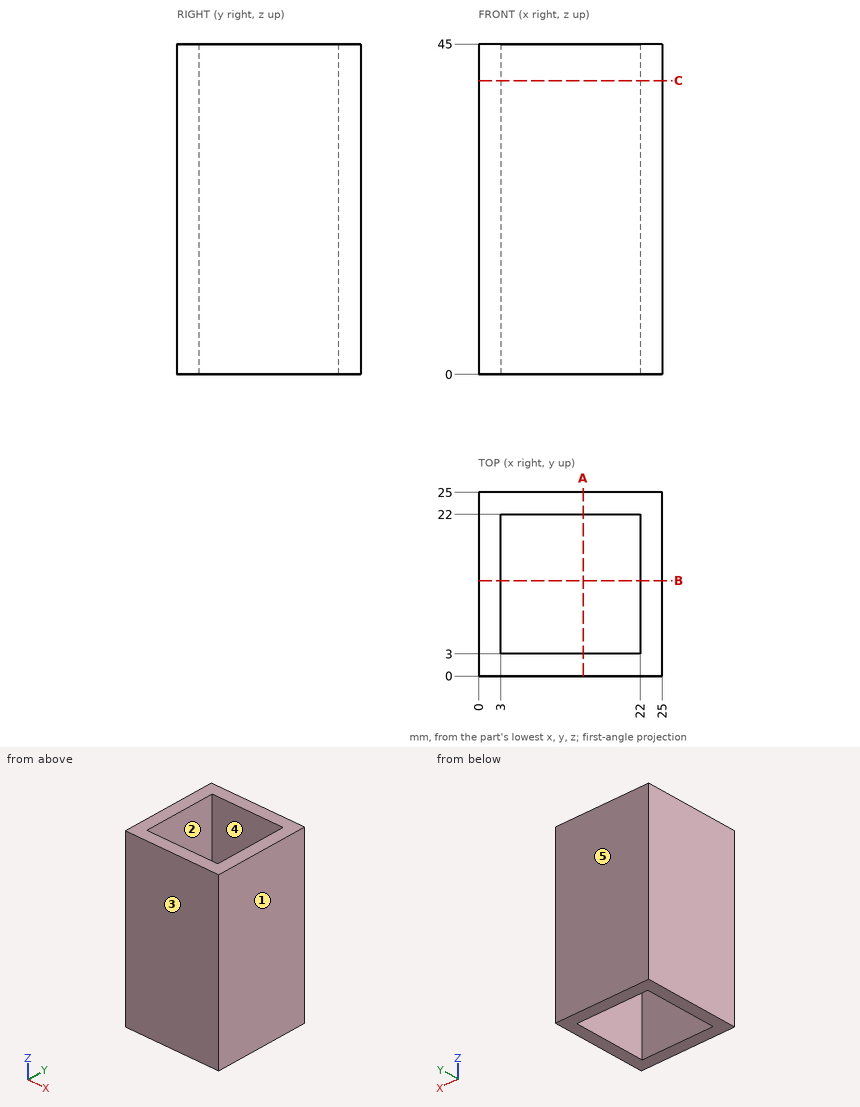
The drawing under review shows one solid part. Ordinate dimensions are in mm from its lowest x, y, z. A direction names the side the tool comes from. Round coordinates to 2 decimals unless told otherwise and drop trailing zeros. Loops run counter-clockwise (first coordinate to the right, second up) from the corner with the lowest first, then second, coordinate; pieces in that order, holes last. Notation, with made-up numbers: (-8, 86.5) - (47, 86.5) arc R37 cw to (47, 122.5) - close; hole circle Ø5 at (-25.75, 62.5). An arc over 180 degrees is marked (long way). One line per question, with ' | ' between items.
1. Draft analysis for pull direction Y (two halves, no side actions). For the marked faces 3, 4 and 5, state which applies: released by +Y, released by -Y, zero draft, split by the parting line, or undercut.
Results are:
face 3: released by -Y | face 4: undercut | face 5: released by +Y
2. For L1, parallel to Y at x = 8.75, z = 25.5, list the stretches that pass through material, from the lowest coordinate up. Write a range as [from, to].
Results are:
L1: y = [0, 3], [22, 25]
3. We need section C-C, the plane z = 40. State the section outline as (x, y) points, and give its area (3 significant figures).
Results are:
outline: (0, 0) - (25, 0) - (25, 25) - (0, 25) - close; hole (3, 3) - (22, 3) - (22, 22) - (3, 22) - close | area: 264 mm²
4. For the marked faces 1 and 2, list the 3-axis set-ups (+Z, -Z, +X, -X, +Y, -Y) from which the entire face can be reached by the end or side of a thin tool; tool diameter is ignored.
Results are:
face 1: +Z, -Z, +X, +Y, -Y | face 2: +Z, -Z
5. We need section A-A, the plane x = 14.25. State the section outline as (y, z) points.
Results are:
outline: (0, 0) - (3, 0) - (3, 45) - (0, 45) - close; (22, 0) - (25, 0) - (25, 45) - (22, 45) - close
